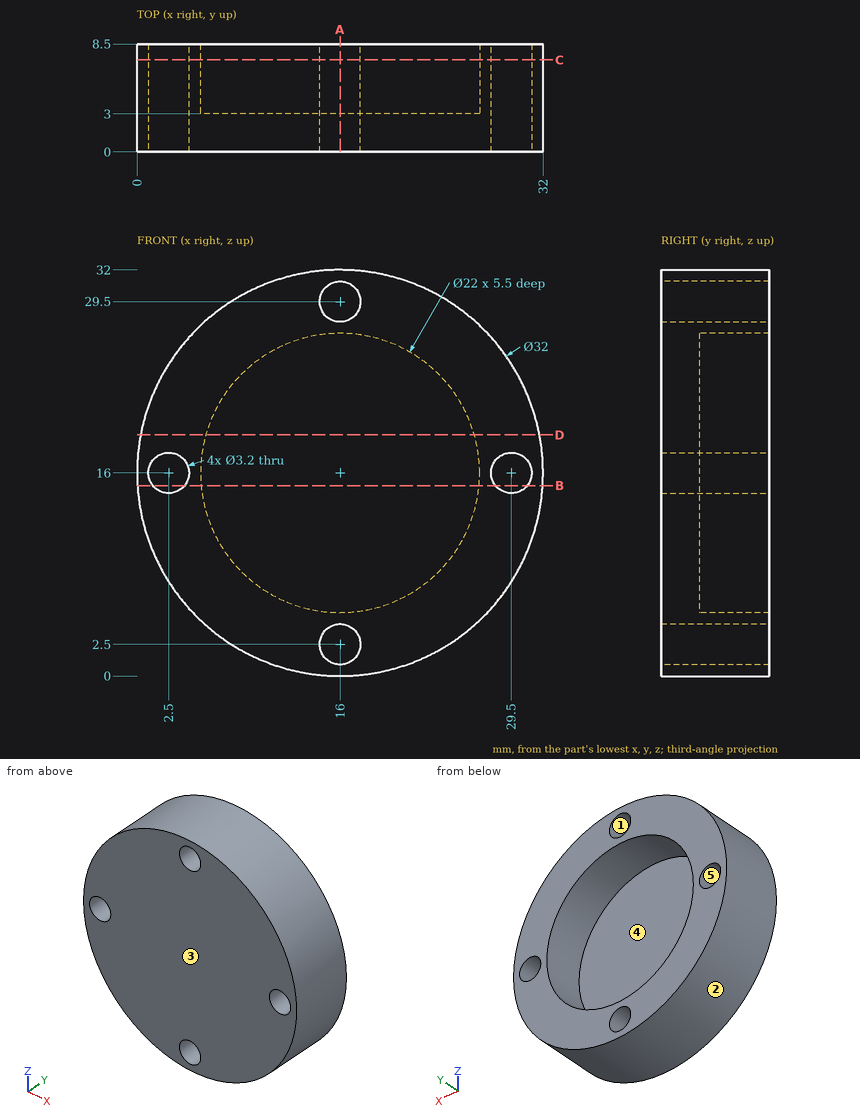
Design review of the part shown in the three views and the two pictorial views. Dimensions are in mm from the part's minimum x, y and z. A direction names the side the tool comes from. Give positions to 0.01 mm unless a question says otherwise; leave off trailing zeros. Write each loop counter-clockwise with the first axis right and the second up, starting at its lowest first coordinate (ties: lowest second). Pieces come first, ordered by that corner, then holes. Notation, with made-up numbers: (15, -9) -> (33, -9) arc R27 ccw to (33, 26) -> close; hole circle Ø1 at (79, -0.5). An arc over 180 degrees is marked (long way). Answer in a Markdown table with one row per item.
1) Add section B-B on z = 15. State the section outline as (x, y) points.
Worked answers:
| item | result |
|---|---|
| outline | (0.03, 0) -> (1.25, 0) -> (1.25, 8.5) -> (0.03, 8.5) -> close; (3.75, 0) -> (28.25, 0) -> (28.25, 8.5) -> (26.95, 8.5) -> (26.95, 3) -> (5.05, 3) -> (5.05, 8.5) -> (3.75, 8.5) -> close; (30.75, 0) -> (31.97, 0) -> (31.97, 8.5) -> (30.75, 8.5) -> close |
2) Add section C-C on y = 7.25. State the section outline as (x, z) points.
Worked answers:
| item | result |
|---|---|
| outline | circle Ø32 at (16, 16); hole circle Ø3.2 at (2.5, 16); hole circle Ø22 at (16, 16); hole circle Ø3.2 at (16, 2.5); hole circle Ø3.2 at (16, 29.5); hole circle Ø3.2 at (29.5, 16) |
3) Tool access review of the marked faces 4 and 5: name each direction out of +Z, -Z, +X, -X, +Y, -Y from which nothing blocks a thin tool from reaching the whole face with its end or side.
Worked answers:
| item | result |
|---|---|
| face 4 | +Y |
| face 5 | +Y, -Y |
4) For L1, parallel to Y at x = 11, z = 22.5; L2, parallel to X at y = 2.25, z = 3.5; L3, parallel to Z at x = 9.5, y = 6.5, list the stretches that pass through material, from the lowest coordinate up. Write a range as [from, to].
Worked answers:
| item | result |
|---|---|
| L1 | [0, 3] |
| L2 | [6.01, 14.75], [17.25, 25.99] |
| L3 | [1.38, 7.13], [24.87, 30.62] |
5) Add section D-D on z = 19. State the section outline as (x, y) points.
Worked answers:
| item | result |
|---|---|
| outline | (0.28, 0) -> (31.72, 0) -> (31.72, 8.5) -> (26.58, 8.5) -> (26.58, 3) -> (5.42, 3) -> (5.42, 8.5) -> (0.28, 8.5) -> close |
6) Add section A-A on x = 16. State the section outline as (y, z) points, plus the area to 3 significant figures.
Worked answers:
| item | result |
|---|---|
| outline | (0, 0) -> (8.5, 0) -> (8.5, 0.9) -> (0, 0.9) -> close; (0, 4.1) -> (8.5, 4.1) -> (8.5, 5) -> (3, 5) -> (3, 27) -> (8.5, 27) -> (8.5, 27.9) -> (0, 27.9) -> close; (0, 31.1) -> (8.5, 31.1) -> (8.5, 32) -> (0, 32) -> close |
| area | 96.6 mm² |
7) Clearance check with flat-ended pins moving along their axes: P1, Ø1, axis at x = 18, y = 7, coming from the -Z side; P2, Ø1.5, axis at y = 6, z = 6, coming from the +X side. State where each tip first meets the part, or that it passes through.
Worked answers:
| item | result |
|---|---|
| P1 | z = 0.07 |
| P2 | x = 29.06 |
8) Mouldability with a two-part tool opening along X and no side actions: class the marked faces 1, 2 and 3 as +X half, -X half, draft (parallel to the pull), parting line (faces both ways), or undercut.
Worked answers:
| item | result |
|---|---|
| face 1 | undercut |
| face 2 | parting line |
| face 3 | draft |
